Verification items for the finished model (mm, model axes). A direction names the side the tool comes from. Give positions to 0.01 mm unless a question says otherwise; leave off trailing zeros. Write each loop counter-clockwise with the first axis right and the second up, starting at its lowest first coordinate (ties: lowest second). Pieces come first, ordered by that corner, then holes. Notation, with made-up numbers: (70.25, 68.25) - (93.25, 68.25) arc R7 ccw to (93.25, 74.25) - close; hole circle Ø4 at (69.25, 24.25). An arc over 180 degrees is marked (long way). Answer as a JSON object with one key per item and string values. Group by question number.
Item 1: Sectioned sample at A-A, the plane x = 0. Record the boundary of the cut face in (y, z) (3 decimals), and give its area (3 significant figures).
Item 2: Scan lines: line 1 along X through (y, z) = (-2, 3); line 2 along Z through (x, y) = (0, -2); line 3 along Z through (x, y) = (4.25, -2). Record each from-to range of solid material in increasing order. Write a range as [from, to].
Item 3: Go/stop test with flat-tipped pins: pin 1 (1.4 mm diameter, centred on x = 0.5, z = 1, fed in from -Y); pin 2 (6 mm diameter, centred on x = 0, z = 33, fed in from -Y); pin 3 (3 mm diameter, centred on x = -0.5, z = 51, fed in from +Y); pin 4 (1 mm diameter, centred on x = 1.5, z = 21, fed in from +Y). Record where each tip stops, or that it passes through.
Item 4: Sectioned sample at B-B, the plane z = 48.5. Record the boundary of the cut face in (x, y), and give its area (3 significant figures).
Item 5: Draft check along Y on faces 1 (the face through (-1.08, 4.88, 2.96)), 2 (the face through (0, 2.5, 2)), 3 (the face through (2.1, -2.1, 0)). Enter one of: +Y half, -Y half, draft (parallel to the pull), parting line (faces both ways), or undercut.
Item 6: Tool access check on faces 4 (the face through (0, 0, 71)), 5 (the face through (-3, 0, 38)), 6 (the face through (-2.175, -1.233, 1.813)). Record the directions out of +Z, -Z, +X, -X, +Y, -Y that give a thin tool (end or side, any length) a straight path to the whole face; none if there is none.
Autodesk Inventor part; units mm, degrees
ref_plane "YZ Plane" through (0, 0, 0) normal (1, 0, 0) x (0, 1, 0)
ref_plane "XZ Plane" through (0, 0, 0) normal (0, 1, 0) x (-1, 0, 0)
ref_plane "XY Plane" through (0, 0, 0) normal (0, 0, 1) x (1, 0, 0)
sketch "Sketch1" plane through (0, 0, 0) normal (0, 0, 1) x (1, 0, 0)
  circle A0 centre (0, 0) radius 5
  dimension "d0" = 10
extrude "Extrusion1" add sketch "Sketch1" along normal blind 6
sketch "Sketch2" plane through (0, 0, 6) normal (0, 0, 1) x (1, 0, 0)
  circle A0 centre (0, 0) radius 3
  dimension "d3" = 6
extrude "Extrusion2" add sketch "Sketch2" along normal blind 65
thread "Thread1"
fillet "Fillet2" radius 0.5 1 edges at (-3, 0, 71)
fillet "Fillet3" radius 0.2 3 edges at (-5, 0, 6) (-3, 0, 6) (-5, 0, 0)
sketch "Sketch5" plane through (0, 0, 0) normal (0, 0, -1) x (-1, 0, 0)
  line L0 (2.8868, 0) -> (1.4434, -2.5)
  line L1 (1.4434, -2.5) -> (-1.4434, -2.5)
  line L2 (-1.4434, -2.5) -> (-2.8868, 0)
  line L3 (-2.8868, 0) -> (-1.4434, 2.5)
  line L4 (-1.4434, 2.5) -> (1.4434, 2.5)
  line L5 (1.4434, 2.5) -> (2.8868, 0)
  point P0 (0, 0)
  point P1 (0, 0)
  dimension "d15" = 5
extrude "Extrusion4" cut sketch "Sketch5" against normal blind 3.7
fillet "Fillet6" radius 0.125 6 edges at (-2.1651, -1.25, 3.7) (0, -2.5, 3.7) (0, 2.5, 3.7) (-2.1651, 1.25, 3.7) (2.1651, -1.25, 3.7) (2.1651, 1.25, 3.7)
fillet "Fillet7" radius 0.1 6 edges at (-2.1651, -1.25, 0) (0, -2.5, 0) (2.1651, -1.25, 0) (2.1651, 1.25, 0) (0, 2.5, 0) (-2.1651, 1.25, 0)
properties part number "MM-MMount_to_Frame-Bolt"
Geometry check:
{
 "1": {"outline": "(-5, 0.2) arc R0.2 ccw to (-4.8, 0) - (-2.6, 0) arc R0.1 ccw to (-2.5, 0.1) - (-2.5, 3.575) arc R0.125 cw to (-2.375, 3.7) - (2.375, 3.7) arc R0.125 cw to (2.5, 3.575) - (2.5, 0.1) arc R0.1 ccw to (2.6, 0) - (4.8, 0) arc R0.2 ccw to (5, 0.2) - (5, 5.8) arc R0.2 ccw to (4.8, 6) - (3.2, 6) arc R0.2 cw to (3, 6.2) - (3, 70.5) arc R0.5 ccw to (2.5, 71) - (-2.5, 71) arc R0.5 ccw to (-3, 70.5) - (-3, 6.2) arc R0.2 cw to (-3.2, 6) - (-4.8, 6) arc R0.2 ccw to (-5, 5.8) - close", "area": "431 mm^2"},
 "2": {"line 1": "[-4.58, -1.73], [1.73, 4.58]", "line 2": "[3.7, 71]", "line 3": "[0, 6]"},
 "3": {"pin 1": "y = -5", "pin 2": "y = -3", "pin 3": "y = 3", "pin 4": "y = 2.83"},
 "4": {"outline": "circle Ø6 at (0, 0)", "area": "28.3 mm^2"},
 "5": {"face 1": "parting line", "face 2": "undercut", "face 3": "draft"},
 "6": {"face 4": "+Z, +X, -X, +Y, -Y", "face 5": "+Z", "face 6": "-Z"}
}
